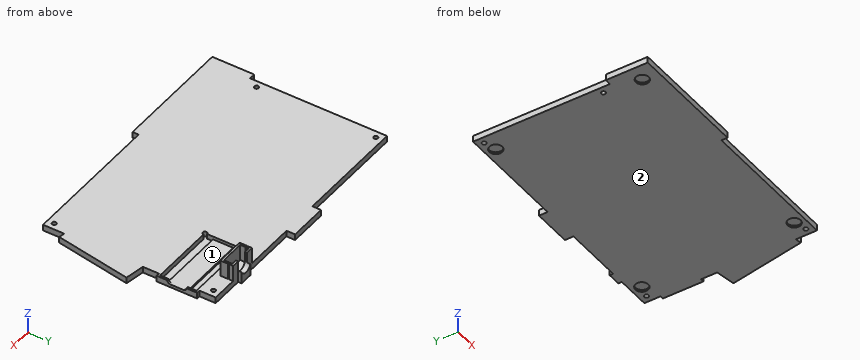
```python
from build123d import *

# Parameters (mm, degrees)
PAD017_DEPTH    = 3
SKETCH041_R     = 1.05
POCKET007_DEPTH = 3.001
PAD018_DEPTH    = 1.7
SKETCH043_W     = 33
SKETCH043_H     = 17.9
POCKET008_DEPTH = 1.5
POCKET009_DEPTH = 2.5
SKETCH045_W     = 6.4
SKETCH045_H     = 7
PAD019_DEPTH    = 1.7
PAD020_DEPTH    = 8
POCKET010_DEPTH = 6.9
SKETCH048_R     = 3.15
POCKET011_DEPTH = 1


with BuildPart() as part:
    # Sketch040 (on Face97 of Binder002) → Pad017 (new body)
    with BuildSketch(Plane.XY.offset(-8)):
        Polygon((-64.45, 24.325), (-64.45, -43.04), (-67.45, -43.04), (-67.45, -63.64), (-8.75, -63.64), (-8.75, -60.64), (61.6428917544, -60.64), (61.6428917544, -50.1977285884), (64.5583406887, -50.7118008964), (71.1743362578, -13.1906255066), (61.6428917544, -11.5099746756), (61.6428917544, 24.325), (9.525, 24.325), (9.525, 28.575), (-9.525, 28.575), (-9.525, 24.325), align=None)
    extrude(amount=-PAD017_DEPTH)

    # Sketch041 (on Face17 of Pad017) → Pocket007 (cut, through all)
    with BuildSketch(Plane.XY.offset(-8)):
        with Locations((-61.15, 21.025)):
            Circle(SKETCH041_R)
        with Locations((-61.15, -37.64)):
            Circle(SKETCH041_R)
        with Locations((58.3428917544, 21.025)):
            Circle(SKETCH041_R)
        with Locations((58.3428917544, -57.34)):
            Circle(SKETCH041_R)
    extrude(amount=-POCKET007_DEPTH, mode=Mode.SUBTRACT)

    # Sketch042 (on Vertex202 of Binder002) → Pad018 (join)
    with BuildSketch(Plane(origin=(61.6428917544, 16.525, -11), x_dir=(0, 1, 0), z_dir=(1, 0, 0))):
        with BuildLine():
            Line((-0.2, 0), (-0.2, 3))
            Line((-0.2, 3), (-5.5, 3))
            Line((-5.5, 2.9), (-5.5, 3))
            ThreePointArc((-6.9, 1.5), (-5.9100505063, 1.9100505063), (-5.5, 2.9))
            Line((-13.4, 1.5), (-6.9, 1.5))
            ThreePointArc((-14.8, 2.9), (-14.3899494937, 1.9100505063), (-13.4, 1.5))
            Line((-14.8, 3), (-14.8, 2.9))
            Line((-20.1, 3), (-14.8, 3))
            Line((-20.1, 3), (-20.1, 0))
            Line((-20.1, 0), (-0.2, 0))
        make_face()
    extrude(amount=PAD018_DEPTH)

    # Sketch043 (on Vertex40 of Pad018) → Pocket008 (cut)
    with BuildSketch(Plane(origin=(63.3428917544, 16.325, -8), x_dir=(1, 0, 0), z_dir=(0, 0, 1))):
        with Locations((-17.5, -9.95)):
            Rectangle(SKETCH043_W, SKETCH043_H)
    extrude(amount=-POCKET008_DEPTH, mode=Mode.SUBTRACT)

    # Sketch044 (on Face4 of Pocket008) → Pocket009 (cut)
    with BuildSketch(Plane.XY.offset(-8)):
        with BuildLine():
            ThreePointArc((30.3428917544, 15.3249996463), (28.6357850983, 16.0321069062), (29.3428917544, 14.325))
            Line((29.3428917544, 14.325), (29.3428917544, 11.3249996463))
            Line((29.3428917544, 11.3249996463), (62.3428917544, 11.3249996463))
            Line((62.3428917544, 11.3249996463), (62.3428917544, 15.3249996463))
            Line((30.3428917544, 15.3249996463), (62.3428917544, 15.3249996463))
        make_face()
        with BuildLine():
            ThreePointArc((29.3428917544, -1.575), (28.6357848482, -3.2821066561), (30.3428917544, -2.5750003537))
            Line((62.3428917544, -2.5750003537), (30.3428917544, -2.5750003537))
            Line((62.3428917544, -2.5750003537), (62.3428917544, 1.4249996463))
            Line((62.3428917544, 1.4249996463), (29.3428917544, 1.4249996463))
            Line((29.3428917544, 1.4249996463), (29.3428917544, -1.575))
        make_face()
    extrude(amount=-POCKET009_DEPTH, mode=Mode.SUBTRACT)

    # Sketch045 (on Vertex102 of Binder002) → Pad019 (join)
    with BuildSketch(Plane(origin=(38.4428917544, 24.325, -11), x_dir=(1, 0, 0), z_dir=(0, -1, 0))):
        with Locations((3.4, 3.5)):
            Rectangle(SKETCH045_W, SKETCH045_H)
    extrude(amount=-PAD019_DEPTH)

    # Sketch046 (on Vertex13 of Pad019) → Pad020 (join)
    with BuildSketch(Plane(origin=(45.0428917544, 24.325, -8), x_dir=(1, 0, 0), z_dir=(0, 0, 1))):
        Polygon((-9.2, -1), (-9.2, -2), (-10.2, -2), (-10.2, 0), (3.8, 0), (3.8, -2), (2.8, -2), (2.8, -1), align=None)
        Polygon((-10.2, -2.5), (-9.2, -2.5), (-9.2, -5.2), (2.8, -5.2), (2.8, -2.5), (3.8, -2.5), (3.8, -6.2), (-10.2, -6.2), align=None)
    extrude(amount=PAD020_DEPTH)

    # Sketch047 (on Face51 of Pad020) → Pocket010 (cut)
    with BuildSketch(Plane(origin=(0, 26.025, 0), x_dir=(-1, 0, 0), z_dir=(0, 1, 0))):
        with BuildLine():
            ThreePointArc((-45.2428917544, -4), (-41.8428917544, -7.4), (-38.4428917544, -4))
            Line((-38.4428917544, 0), (-38.4428917544, -4))
            Line((-45.2428917544, 0), (-38.4428917544, 0))
            Line((-45.2428917544, -4), (-45.2428917544, 0))
        make_face()
    extrude(amount=-POCKET010_DEPTH, mode=Mode.SUBTRACT)

    # Sketch048 (on Face5 of Pocket010) → Pocket011 (cut)
    with BuildSketch(Plane(origin=(0, 0, -11), x_dir=(1, 0, 0), z_dir=(0, 0, -1))):
        with Locations((-59.45, 55.64)):
            Circle(SKETCH048_R)
        with Locations((52.3428917545, 55.64)):
            Circle(SKETCH048_R)
        with Locations((-55.15, -19.325)):
            Circle(SKETCH048_R)
        with Locations((52.3428917545, -19.325)):
            Circle(SKETCH048_R)
    extrude(amount=-POCKET011_DEPTH, mode=Mode.SUBTRACT)


solid = part.part
```
Check sheet for the modelled part. Datum: model origin and axes. Units: mm. Face numbers are marked on the shaded views. Coordinates: 2 decimals unless noted, no trailing zeros. Write each loop counter-clockwise with the first axis right and the second up, starting at its lowest first coordinate (ties: lowest second). Pieces come first, ordered by that corner, then holes. Notation, with made-up numbers: M 5,84.5 L 28,84.5 A23 cw 28,113.5 Z; hole C -34.75,-39 d1. An arc over 180 degrees is marked long. Use one line per item in the form item = value.
Item 1: Release check for a two-part mould opening along Y. For the marked faces 1 and 2 record: pulls with the +Y half, pulls with the -Y half, needs draft (parallel to the pull), parting line crosses it, or undercut.
Answer below:
face_1 = undercut
face_2 = needs draft
Item 2: Sectioned sample at B-B, the plane x = -27. Record the cut outline in (y, z) (3 decimals).
Answer below:
outline = M -63.64,-11 L 24.325,-11 L 24.325,-8 L -63.64,-8 Z
Item 3: Material ranges on L1, parallel to X at y = -55.64, z = -10.5; L2, parallel to Y at x = 38, z = -0.25 (3 decimals); L3, parallel to Z at x = 60, y = 6.5, recorded low to high. Write a range as from..to.
Answer below:
L1 = -67.45..-62.6, -56.3..49.19, 55.49..61.64
L2 = 18.125..19.125, 23.325..24.325
L3 = -11..-9.5
Item 4: Sectioned sample at A-A, the plane y = -7. Record the cut outline in (x, z).
Answer below:
outline = M -64.45,-11 L 61.64,-11 L 61.64,-8 L -64.45,-8 Z
Item 5: Gauge pin test, flat ends, axial feed: pin 1 Ø0.8 at (y, z) = (24, -3) entering from -X; pin 2 Ø1.5 at (x, y) = (-38.5, -47) entering from +Z; pin 3 Ø1.5 at (x, z) = (34.5, -6.5) entering from +Y (3 decimals); pin 4 Ø2 at (x, z) = (-50, -5.5) entering from +Y (3 decimals). Record the tip position at first contact, or that the pin passes through.
Answer below:
pin_1 = 34.84
pin_2 = -8
pin_3 = 24.325
pin_4 = through
